The listing builds one solid part. Answer for the finished solid, in the listing's coordinates (mm). Face numbers are marked on the shaded views. Give positions to 0.01 mm unless a question says otherwise; leave off trailing zeros. Loops run counter-clockwise (first coordinate to the right, second up) from the corner with the lowest first, then second, coordinate; pieces in that order, holes last. Notation, with made-up numbers: (0, -32.5) - (29, -32.5) arc R15 ccw to (29, -27.5) - close; hole circle Ø2 at (-40, -14.75). An arc over 180 degrees is marked (long way). Write item = value, one per line. Start each with the question number.
1) Flat-ended cylindrical pins translate along their axes: P1, Ø1, axis at y = 6, z = 6, coming from the +X side; P2, Ø0.5, axis at x = 73.5, z = 5, coming from the -Y side; P3, Ø0.5, axis at x = 6.5, z = 7, coming from the -Y side. Find the tip coordinate at first contact, or state that the pin passes through.
2) Consider probe 1 along X at (y, z) = (5.25, 6.75); probe 2 along X at (y, z) = (5.75, 9.75); probe 3 along Y at (x, z) = (48, 5.5). Determine where each line is inside the solid, lowest interval first.
3) The part is cut by section A-A on y = 5.75. Write down the section's boundary in (x, z).
4) The mould has two halves that part along X. Classify the marked faces 1, 2, 3 and 4: +X half, -X half, draft (parallel to the pull), parting line (faces both ways), or undercut.
5) The part is cut by section C-C on x = 54. Write down the section's boundary in (y, z).
6) The part is cut by section B-B on x = 76. Write down the section's boundary in (y, z), plus the area to 3 significant figures.
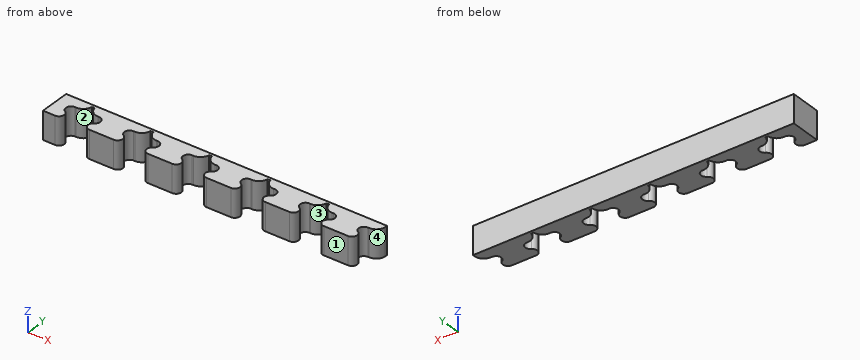
Autodesk Inventor part; units mm, degrees
ref_plane "YZ Plane" through (0, 0, 0) normal (1, 0, 0) x (0, 1, 0)
ref_plane "XZ Plane" through (0, 0, 0) normal (0, 1, 0) x (-1, 0, 0)
ref_plane "XY Plane" through (0, 0, 0) normal (0, 0, 1) x (1, 0, 0)
sketch "Sketch1" plane through (0, 0, 0) normal (0, 0, 1) x (1, 0, 0)
  line L0 (0, 0) -> (21, 0)
  line L1 (21, 0) -> (21, 11)
  line L2 (21, 11) -> (0, 11)
  line L3 (0, 11) -> (0, 0)
  dimension "d0" = 21
  dimension "d1" = 11
extrude "Extrusion1" add sketch "Sketch1" along normal blind 10
sketch "Sketch2" plane through (0, 0, 10) normal (0, 0, 1) x (1, 0, 0)
  line L0 (0, 0) -> (21, 0)
  arc A0 (4.3181, 0) -> (5.25, 3.5) centre (4.3181, 1.8741) ccw
  arc A1 (6.1819, 7) -> (5.25, 3.5) centre (6.1819, 5.1259) ccw
  arc A2 (15.75, 3.5) -> (16.6819, 0) centre (16.6819, 1.8741) ccw
  arc A3 (15.75, 3.5) -> (14.8181, 7) centre (14.8181, 5.1259) ccw
  line L1 (6.1819, 7) -> (14.8181, 7)
  line L2 (21, 11) -> (0, 11)
  line L3 (4.3181, 1.8741) -> (6.1819, 5.1259) construction
  line L4 (16.6819, 1.8741) -> (14.8181, 5.1259) construction
  line L5 (0, 11) -> (0, 0) construction
  line L6 (21, 0) -> (21, 11) construction
  point P0 (10.5, 7)
  point P1 (15.75, 3.5)
  dimension "d7" = 10.5
  dimension "d9" = 7
  dimension "d13" = 10.5
extrude "Extrusion2" cut sketch "Sketch2" against normal through all
sketch "Sketch3" plane through (0, 0, 10) normal (0, 0, 1) x (1, 0, 0)
  line L0 (21, 11) -> (0, 11)
  line L1 (14.8181, 7) -> (6.1819, 7)
  arc A0 (6.6147, 7) -> (10, 10) centre (6.6147, 10.41) ccw
  arc A1 (11, 10) -> (14.3853, 7) centre (14.3853, 10.41) ccw
  line L2 (10, 10) -> (11, 10)
  line L3 (6.1819, 7) -> (14.8181, 7)
  line L4 (10.5, 10) -> (10.5, 11) construction
  point P0 (0, 0)
  dimension "d15" = 1
  dimension "d16" = 1
extrude "Extrusion3" cut sketch "Sketch3" against normal through all
pattern_linear "Rectangular Pattern1" count 6 spacing 21 along (1, 0, 0)
sketch "Sketch4" plane through (0, 0, 10) normal (0, 0, 1) x (1, 0, 0)
  line L0 (115, 10) -> (116, 10)
  line L1 (115, 10) -> (115, 11)
  line L2 (126, 11) -> (0, 11)
  line L3 (121.6819, 0) -> (126, 0)
  line L4 (121.6819, 0) -> (126, 0)
  line L5 (126, 0) -> (126, 11)
  line L6 (126, 0) -> (126, 11)
  line L7 (126, 11) -> (115, 11)
  arc A0 (116, 10) -> (119.3853, 7) centre (119.3853, 10.41) ccw
  line L8 (115, 10) -> (116, 10)
  line L9 (119.3853, 7) -> (119.8181, 7)
  arc A1 (116, 10) -> (119.3853, 7) centre (119.3853, 10.41) ccw
  arc A2 (120.75, 3.5) -> (119.8181, 7) centre (119.8181, 5.1259) ccw
  line L10 (119.3853, 7) -> (119.8181, 7)
  arc A3 (120.75, 3.5) -> (119.8181, 7) centre (119.8181, 5.1259) ccw
  arc A4 (120.75, 3.5) -> (121.6819, 0) centre (121.6819, 1.8741) ccw
  arc A5 (120.75, 3.5) -> (121.6819, 0) centre (121.6819, 1.8741) ccw
  point P0 (0, 0)
extrude "Extrusion4" cut sketch "Sketch4" against normal through all
properties part number "Zipperteethv3"
Answer below:
q1.P1 = 109.91
q1.P2 = 10
q1.P3 = 7
q2.probe_1 = 0 to 4.31, 16.69 to 25.31, 37.69 to 46.31, 58.69 to 67.31, 79.69 to 88.31, 100.69 to 109.31
q2.probe_2 = 0 to 4.41, 16.59 to 25.41, 37.59 to 46.41, 58.59 to 67.41, 79.59 to 88.41, 100.59 to 109.41
q2.probe_3 = 1.05 to 2.7, 6.99 to 11
q3.outline = (0, 0) - (4.41, 0) - (4.41, 10) - (0, 10) - close; (16.59, 0) - (25.41, 0) - (25.41, 10) - (16.59, 10) - close; (37.59, 0) - (46.41, 0) - (46.41, 10) - (37.59, 10) - close; (58.59, 0) - (67.41, 0) - (67.41, 10) - (58.59, 10) - close; (79.59, 0) - (88.41, 0) - (88.41, 10) - (79.59, 10) - close; (100.59, 0) - (109.41, 0) - (109.41, 10) - (100.59, 10) - close
q4.face_1 = draft
q4.face_2 = undercut
q4.face_3 = undercut
q4.face_4 = +X half
q5.outline = (7.97, 0) - (11, 0) - (11, 10) - (7.97, 10) - close
q6.outline = (7.29, 0) - (11, 0) - (11, 10) - (7.29, 10) - close
q6.area = 37.1 mm2
